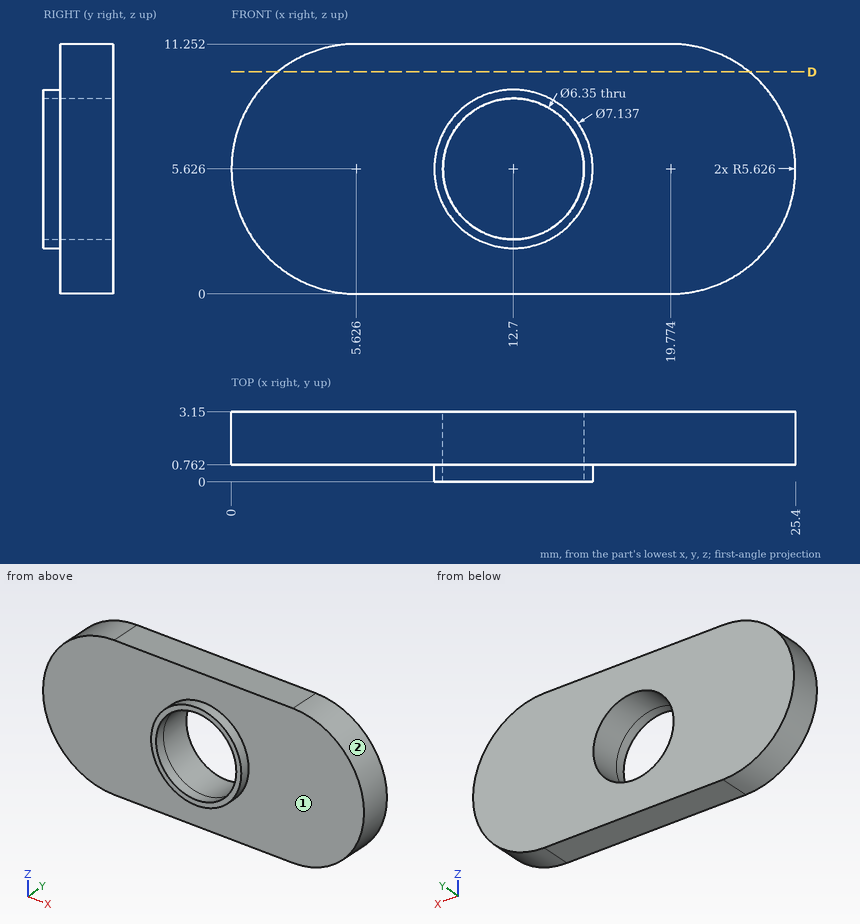
Could you check a few things on this drawing? It's one solid part, dimensions in mm from its lowest x, y, z. A direction names the side the tool comes from. Give positions to 0.01 mm unless a question says otherwise; leave off trailing zeros. Loops run counter-clockwise (first coordinate to the right, second up) from the corner with the lowest first, then second, coordinate; pieces in that order, holes last. Notation, with made-up numbers: M 68,-18.5 L 118,-18.5 A24 cw 118,20.5 Z; hole C 61.5,49 d6. An arc over 180 degrees is marked long. Return JSON: item names as keys, results as strings.
Item 1: On a 3-axis mill with a long thin cutter (end or side, diameter ignored), from which of +Z, -Z, +X, -X, +Y, -Y can I reach the whole of each face in a straight line? I mean the marked faces 1 and 2. Say none if no direction works.
A:
{"face 1": "-Y", "face 2": "+X, +Y, -Y"}
Item 2: Please list where these lines run through material, in increasing order: line 1 (Z direction, x = 12.7, y = 0.3) (1 decimal); line 2 (Y direction, x = 12.25, z = 10.5); line 3 (Z direction, x = 12.7, y = 2.6).
A:
{"line 1": "z = 2.1 to 2.5, 8.8 to 9.2", "line 2": "y = 0.76 to 3.15", "line 3": "z = 0 to 2.45, 8.8 to 11.25"}
Item 3: Imagine slicing it at D-D on z = 10. List the corners of the cut face in (x, y) for me.
A:
{"outline": "M 2.09,0.76 L 23.31,0.76 L 23.31,3.15 L 2.09,3.15 Z"}
Item 4: I'm going to push a flat-ended pin straight in: pin 1 Ø5.5 at (x, z) = (12.7, 5.63) entering from -Y. Where does the tip first touch, or does it pass through?
A:
{"pin 1": "passes through"}
